Check sheet for the modelled part. Datum: model origin and axes. Units: mm. Face numbers are marked on the shaded views. Round coordinates to 2 decimals unless told otherwise and drop trailing zeros. Write each loop counter-clockwise with the first axis right and the second up, starting at its lowest first coordinate (ties: lowest second). Pieces come first, ordered by that corner, then holes. Notation, with made-up numbers: (-26, 50) - (18, 50) arc R15 ccw to (18, 66) - close; hole circle Ø8 at (-28.75, 5.5). An arc over 180 degrees is marked (long way). Answer as a JSON object with one key per item and string values. Group by question number.
Item 1: Release check for a two-part mould opening along X. For the marked faces 1, 2 and 3 record: pulls with the +X half, pulls with the -X half, needs draft (parallel to the pull), parting line crosses it, or undercut.
Item 2: Sectioned sample at C-C on y = 1.75. Count the separate pieces of the cut face and the enclosed holes in it, plus the area to 3 significant figures.
Item 3: Sectioned sample at D-D on z = 5.75. Record the boundary of the cut face in (x, y) (1 decimal), plus the area to 3 significant figures.
Item 4: Gauge pin test, flat end, axial feed: P1, Ø5.5, axis at x = 0, z = -9.525, coming from the +Y side (3 decimals). Record the tip position at first contact, or that the pin passes through.
Item 5: Sectioned sample at A-A on x = 0. Record the boundary of the cut face in (y, z) (1 decimal), plus the area to 3 significant figures.
Item 6: Sectioned sample at B-B on z = 0. Record the boundary of the cut face in (x, y) (1 decimal).
Item 7: Thickness scan on line 1 (Z direction, x = -8.25, y = 0.45); line 2 (Z direction, x = -1, y = 3); line 3 (X direction, y = 2.9, z = 4). Record the ranges inside material, lowest first.
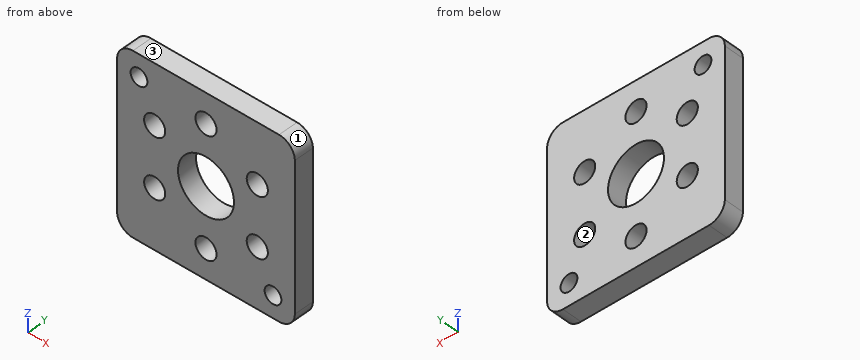
```python
from build123d import *

# Parameters (mm, degrees)
SKETCH1_W             = 28.575
SKETCH1_H             = 28.575
BOSS_EXTRUDE1_DEPTH   = 3.175
M3_CLEARANCE_HOLE1_D  = 3.4
SKETCH2_R             = 4.5
CUT_EXTRUDE2_DEPTH    = 21.453506729
CIRPATTERN1_COUNT     = 6
F_6_32_TAPPED_HOLE1_D = 2.7051
FILLET1_R             = 2.54


with BuildPart() as part:
    # Sketch1 → Boss-Extrude1 (new body)
    with BuildSketch(Plane(origin=(0, 0, 0), x_dir=(1, 0, 0), z_dir=(0, 1, 0))):
        Rectangle(SKETCH1_W, SKETCH1_H)
    extrude(amount=BOSS_EXTRUDE1_DEPTH)

    # M3 Clearance Hole1 (through all)
    with Locations(Plane(origin=(0, 3.175, 0), x_dir=(1, 0, 0), z_dir=(0, 1, 0))):
        with Locations((0, 9.525)):
            m3_clearance_hole1 = Hole(M3_CLEARANCE_HOLE1_D / 2)

    # Sketch2 → Cut-Extrude2 (cut, through all)
    with BuildSketch(Plane(origin=(0, 3.175, 0), x_dir=(1, 0, 0), z_dir=(0, 1, 0))):
        with Locations(Location((0, 0, 0), (0, 0, 270))):
            Circle(SKETCH2_R)
    extrude(amount=-CUT_EXTRUDE2_DEPTH, mode=Mode.SUBTRACT)

    # CirPattern1: M3 Clearance Hole1 ×6 about axis
    cirpattern1_axis = Axis((0, 0, 0), (0, 1, 0))
    for i in range(1, CIRPATTERN1_COUNT):
        add(m3_clearance_hole1.rotate(cirpattern1_axis, i * 360 / CIRPATTERN1_COUNT), mode=Mode.SUBTRACT)

    # #6-32 Tapped Hole1 (through all)
    with Locations(Plane(origin=(0, 3.175, 0), x_dir=(1, 0, 0), z_dir=(0, 1, 0))):
        with Locations((10.776307345, 10.776307345), (-10.776307345, -10.776307345)):
            Hole(F_6_32_TAPPED_HOLE1_D / 2)

    # Fillet1
    fillet1_edges = [part.edges().sort_by_distance(p)[0] for p in [
        (14.2875, 1.5875, 14.2875),
        (-14.2875, 1.5875, 14.2875),
        (-14.2875, 1.5875, -14.2875),
        (14.2875, 1.5875, -14.2875),
    ]]
    fillet(fillet1_edges, radius=FILLET1_R)


solid = part.part
```
Completed:
{
 "1": {"face 1": "pulls with the +X half", "face 2": "undercut", "face 3": "needs draft"},
 "2": {"separate pieces": "1", "enclosed holes": "9", "area": "681 mm²"},
 "3": {"outline": "(-14.3, 0) - (-9.6, 0) - (-9.6, 3.2) - (-14.3, 3.2) - close; (-6.9, 0) - (6.9, 0) - (6.9, 3.2) - (-6.9, 3.2) - close; (9.6, 0) - (14.3, 0) - (14.3, 3.2) - (9.6, 3.2) - close", "area": "73.2 mm²"},
 "4": {"P1": "y = 3.175"},
 "5": {"outline": "(0, -14.3) - (3.2, -14.3) - (3.2, -11.2) - (0, -11.2) - close; (0, -7.8) - (3.2, -7.8) - (3.2, -4.5) - (0, -4.5) - close; (0, 4.5) - (3.2, 4.5) - (3.2, 7.8) - (0, 7.8) - close; (0, 11.2) - (3.2, 11.2) - (3.2, 14.3) - (0, 14.3) - close", "area": "40.6 mm²"},
 "6": {"outline": "(-14.3, 0) - (-4.5, 0) - (-4.5, 3.2) - (-14.3, 3.2) - close; (4.5, 0) - (14.3, 0) - (14.3, 3.2) - (4.5, 3.2) - close"},
 "7": {"line 1": "-14.29 to -6.46, -3.06 to 3.06, 6.46 to 14.29", "line 2": "-14.29 to -10.9, -8.15 to -4.39, 4.39 to 8.15, 10.9 to 14.29", "line 3": "-14.29 to -9.77, -6.73 to -2.06, 2.06 to 6.73, 9.77 to 14.29"}
}
